Can you work these out from the model? Positions are in its coordinate system, mm. A direction names the side the tool comes from. Give positions to 0.01 mm unless a question says otherwise; leave off trailing zeros. Write each loop counter-clockwise with the first axis right and the second up, starting at its lowest first coordinate (ties: lowest second). Pieces come first, ordered by that corner, then holes.
```python
from build123d import *

# Parameters (mm, degrees)
PAD_DEPTH       = 18
POCKET_DEPTH    = 16
POCKET001_DEPTH = 5
POCKET002_DEPTH = 5


with BuildPart() as part:
    # Sketch → Pad (new body)
    with BuildSketch(Plane.XY):
        with BuildLine():
            Line((-13.5, -16.5), (13.5, -16.5))
            ThreePointArc((13.5, -16.5), (18.449747, -14.449747), (20.5, -9.5))
            Line((20.5, -9.5), (20.5, 9.5))
            ThreePointArc((20.5, 9.5), (18.449747, 14.449747), (13.5, 16.5))
            Line((13.5, 16.5), (-13.5, 16.5))
            ThreePointArc((-13.5, 16.5), (-18.449747, 14.449747), (-20.5, 9.5))
            Line((-20.5, 9.5), (-20.5, -9.5))
            ThreePointArc((-20.5, -9.5), (-18.449747, -14.449747), (-13.5, -16.5))
        make_face()
    extrude(amount=PAD_DEPTH)

    # Sketch001 (on Face10 of Pad) → Pocket (cut)
    with BuildSketch(Plane.XY.offset(18)):
        with BuildLine():
            Line((-19, 11.5), (-19, -11.5))
            ThreePointArc((-19, -11.5), (-17.828427, -14.328427), (-15, -15.5))
            Line((-15, -15.5), (15, -15.5))
            ThreePointArc((15, -15.5), (17.828427, -14.328427), (19, -11.5))
            Line((19, -11.5), (19, 11.5))
            ThreePointArc((19, 11.5), (17.828427, 14.328427), (15, 15.5))
            Line((15, 15.5), (-15, 15.5))
            ThreePointArc((-15, 15.5), (-17.828427, 14.328427), (-19, 11.5))
        make_face()
    extrude(amount=-POCKET_DEPTH, mode=Mode.SUBTRACT)

    # Sketch002 (on Face1 of Pocket) → Pocket001 (cut)
    with BuildSketch(Plane.XZ.offset(16.5)):
        with BuildLine():
            Line((-6, 18), (-6, 15))
            ThreePointArc((-6, 15), (-5.414214, 13.585786), (-4, 13))
            Line((-4, 13), (2, 13))
            ThreePointArc((2, 13), (3.414214, 13.585786), (4, 15))
            Line((4, 15), (4, 18))
            ThreePointArc((4, 18), (3.414214, 19.414214), (2, 20))
            Line((2, 20), (-4, 20))
            ThreePointArc((-4, 20), (-5.414214, 19.414214), (-6, 18))
        make_face()
    extrude(amount=-POCKET001_DEPTH, mode=Mode.SUBTRACT)

    # Sketch003 (on Face13 of Pocket001) → Pocket002 (cut)
    with BuildSketch(Plane(origin=(0, 16.5, 0), x_dir=(-1, 0, 0), z_dir=(0, 1, 0))):
        with BuildLine():
            Line((-13, 18), (-13, 14))
            ThreePointArc((-13, 14), (-12.414214, 12.585786), (-11, 12))
            Line((-11, 12), (9, 12))
            ThreePointArc((9, 12), (10.414214, 12.585786), (11, 14))
            Line((11, 14), (11, 18))
            ThreePointArc((11, 18), (10.414214, 19.414214), (9, 20))
            Line((9, 20), (-11, 20))
            ThreePointArc((-11, 20), (-12.414214, 19.414214), (-13, 18))
        make_face()
    extrude(amount=-POCKET002_DEPTH, mode=Mode.SUBTRACT)


solid = part.part
```
1) Suppose I cut it at A-A on z = 8.75. Write out the boundary of the cut face in (x, y).
Values follow:
outline: (-20.5, -9.5) arc R7 ccw to (-13.5, -16.5) - (13.5, -16.5) arc R7 ccw to (20.5, -9.5) - (20.5, 9.5) arc R7 ccw to (13.5, 16.5) - (-13.5, 16.5) arc R7 ccw to (-20.5, 9.5) - close; hole (-19, -11.5) arc R4 ccw to (-15, -15.5) - (15, -15.5) arc R4 ccw to (19, -11.5) - (19, 11.5) arc R4 ccw to (15, 15.5) - (-15, 15.5) arc R4 ccw to (-19, 11.5) - close
2) For pin 1 Ø1 at (x, y) = (12.5, 6.5) entering from +Z; pin 2 Ø0.8 at (y, z) = (16, 16.5) entering from -X; pin 3 Ø0.8 at (x, y) = (-2.5, -16) entering from +Z, each with a flat end and sliding along its axis, tell me the tip position at first contact or that it passes through.
Values follow:
pin 1: stops at z = 2
pin 2: stops at x = -16.93
pin 3: stops at z = 13
3) If we mould it in two halves opening along Y, with no side actions, what happens to faces 5 (the face through (18.5, 14.4, 8.9)), 6 (the face through (12.43, 16.01, 12.6)), 7 (the face through (0, 0, 2))? For each: +Y half, -Y half, draft (parallel to the pull), parting line (faces both ways), or undercut.
Values follow:
face 5: +Y half
face 6: draft
face 7: undercut
4) For faces 1 (the face through (-18.4, 14.5, 8.9)), 2 (the face through (-1, -16, 13)), 3 (the face through (0, -15.5, 10)), 4 (the face through (-10.4, 16.01, 12.57)), which set-ups out of +Z, -Z, +X, -X, +Y, -Y let a thin tool reach every point of the face, with its end or its side?
Values follow:
face 1: +Z, -Z, -X, +Y
face 2: +Z, +Y, -Y
face 3: +Z
face 4: +Z, +Y
5) Suppose I cut it at D-D on y = 8. Write out the boundary of the cut face in (x, z).
Values follow:
outline: (-20.5, 0) - (20.5, 0) - (20.5, 18) - (19, 18) - (19, 2) - (-19, 2) - (-19, 18) - (-20.5, 18) - close
6) Please list where these lines run through material, in increasing order: L1, parallel to X at y = -7, z = 13.5; L2, parallel to Y at x = 11, z = 7.25; L3, parallel to Z at x = -1.5, y = 12.
Values follow:
L1: x = -20.5 to -19, 19 to 20.5
L2: y = -16.5 to -15.5, 15.5 to 16.5
L3: z = 0 to 2
7) Suppose I cut it at C-C on x = -13. Write out the boundary of the cut face in (y, z).
Values follow:
outline: (-16.5, 0) - (16.5, 0) - (16.5, 18) - (15.5, 18) - (15.5, 2) - (-15.5, 2) - (-15.5, 18) - (-16.5, 18) - close
8) Suppose I cut it at B-B on z = 16.25. Write out the boundary of the cut face in (x, y), plus the area to 3 significant figures.
Values follow:
outline: (-20.5, -9.5) arc R7 ccw to (-13.5, -16.5) - (-6, -16.5) - (-6, -15.5) - (-15, -15.5) arc R4 cw to (-19, -11.5) - (-19, 11.5) arc R4 cw to (-15, 15.5) - (-11, 15.5) - (-11, 16.5) - (-13.5, 16.5) arc R7 ccw to (-20.5, 9.5) - close; (4, -16.5) - (13.5, -16.5) arc R7 ccw to (20.5, -9.5) - (20.5, 9.5) arc R7 ccw to (13.5, 16.5) - (13, 16.5) - (13, 15.5) - (15, 15.5) arc R4 cw to (19, 11.5) - (19, -11.5) arc R4 cw to (15, -15.5) - (4, -15.5) - close
area: 113 mm2
